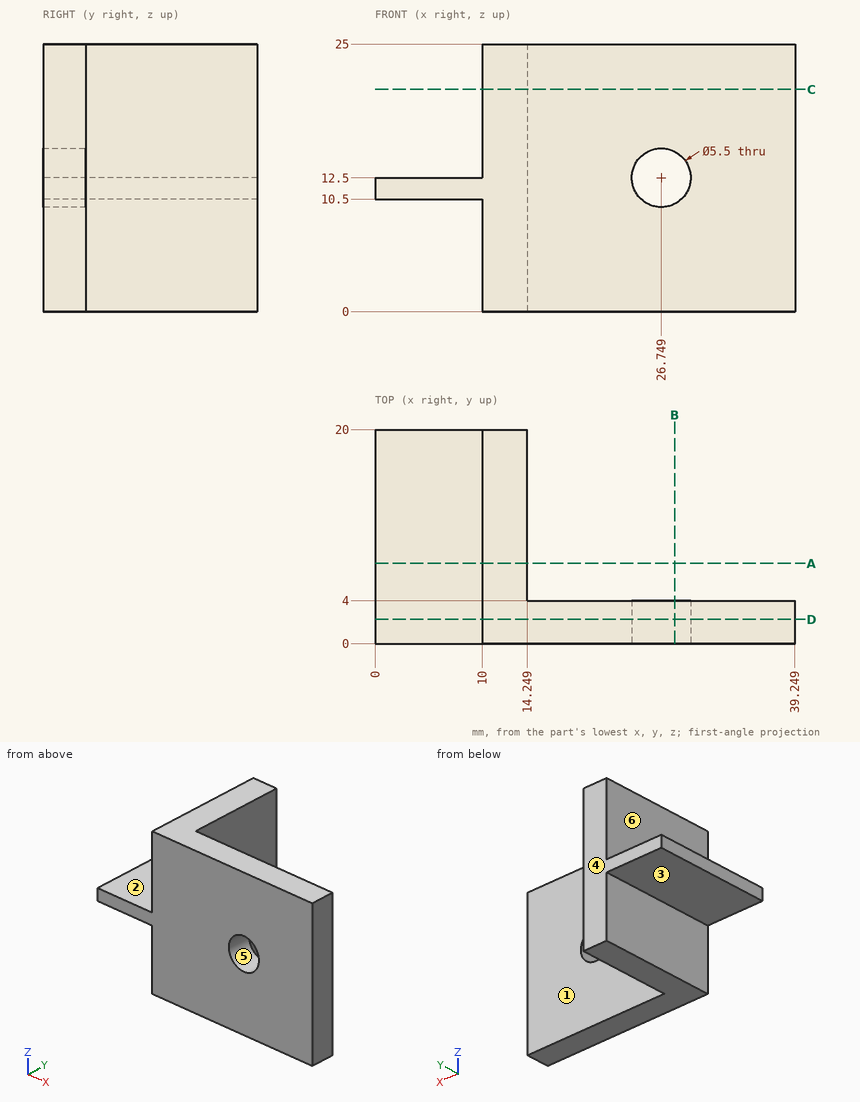
Design review of the part shown in the three views and the two pictorial views. Dimensions are in mm from the part's minimum x, y and z. A direction names the side the tool comes from. Round coordinates to 2 decimals unless told otherwise and drop trailing zeros. Loops run counter-clockwise (first coordinate to the right, second up) from the corner with the lowest first, then second, coordinate; pieces in that order, holes last. Notation, with made-up numbers: (-34, 21.25) -> (-5, 21.25) arc R20 ccw to (-5, 41.25) -> close; hole circle Ø11 at (82, 47). An arc over 180 degrees is marked (long way). Return JSON: item names as keys, results as strings.
(1) Add section A-A on y = 7.5. Write out the cut boundary in (x, z).
Solved:
{"outline": "(0, 10.5) -> (10, 10.5) -> (10, 0) -> (14.25, 0) -> (14.25, 25) -> (10, 25) -> (10, 12.5) -> (0, 12.5) -> close"}
(2) Add section D-D on y = 2.25. Write out the cut boundary in (x, z).
Solved:
{"outline": "(0, 10.5) -> (10, 10.5) -> (10, 0) -> (39.25, 0) -> (39.25, 25) -> (10, 25) -> (10, 12.5) -> (0, 12.5) -> close; hole circle Ø5.5 at (26.75, 12.5)"}
(3) Add section C-C on z = 20.75. Write out the cut boundary in (x, y), plus the area to 3 significant figures.
Solved:
{"outline": "(10, 0) -> (39.25, 0) -> (39.25, 4) -> (14.25, 4) -> (14.25, 20) -> (10, 20) -> close", "area": "185 mm2"}
(4) For line 1 (X direction, y = 6.5, z = 9.5); line 2 (X direction, y = 2.5, z = 16.25); line 3 (Z direction, x = 8, y = 9.25), list the stretches that pass through material, from the lowest coordinate up.
Solved:
{"line 1": "10 to 14.25", "line 2": "10 to 39.25", "line 3": "10.5 to 12.5"}
(5) For the marked faces 1, 2 and 3, list the 3-axis set-ups (+Z, -Z, +X, -X, +Y, -Y) from which the entire face can be reached by the end or side of a thin tool; tool diameter is ignored.
Solved:
{"face 1": "+Z, -Z, +X, +Y", "face 2": "+Z, -X, +Y, -Y", "face 3": "-Z, -X, +Y, -Y"}
(6) The part is to be moulded in two halves that separate along X. For the marked faces 4, 5 and 6, say which applies: released by +X, released by -X, zero draft, split by the parting line, or undercut.
Solved:
{"face 4": "zero draft", "face 5": "undercut", "face 6": "released by -X"}
(7) Add section B-B on x = 28. Write out the cut boundary in (y, z).
Solved:
{"outline": "(0, 0) -> (4, 0) -> (4, 10.05) -> (0, 10.05) -> close; (0, 14.95) -> (4, 14.95) -> (4, 25) -> (0, 25) -> close"}
(8) For pin 1 (5 mm diameter, centred on x = 4, y = 12, fed in from +Z); pin 2 (6 mm diameter, centred on y = 9.5, z = 18, fed in from -X); pin 3 (8 mm diameter, centred on y = 13.5, z = 21.5, fed in from +X), all flat-tipped, find the tip position at first contact; note any pin that passes through.
Solved:
{"pin 1": "z = 12.5", "pin 2": "x = 10", "pin 3": "x = 14.25"}
